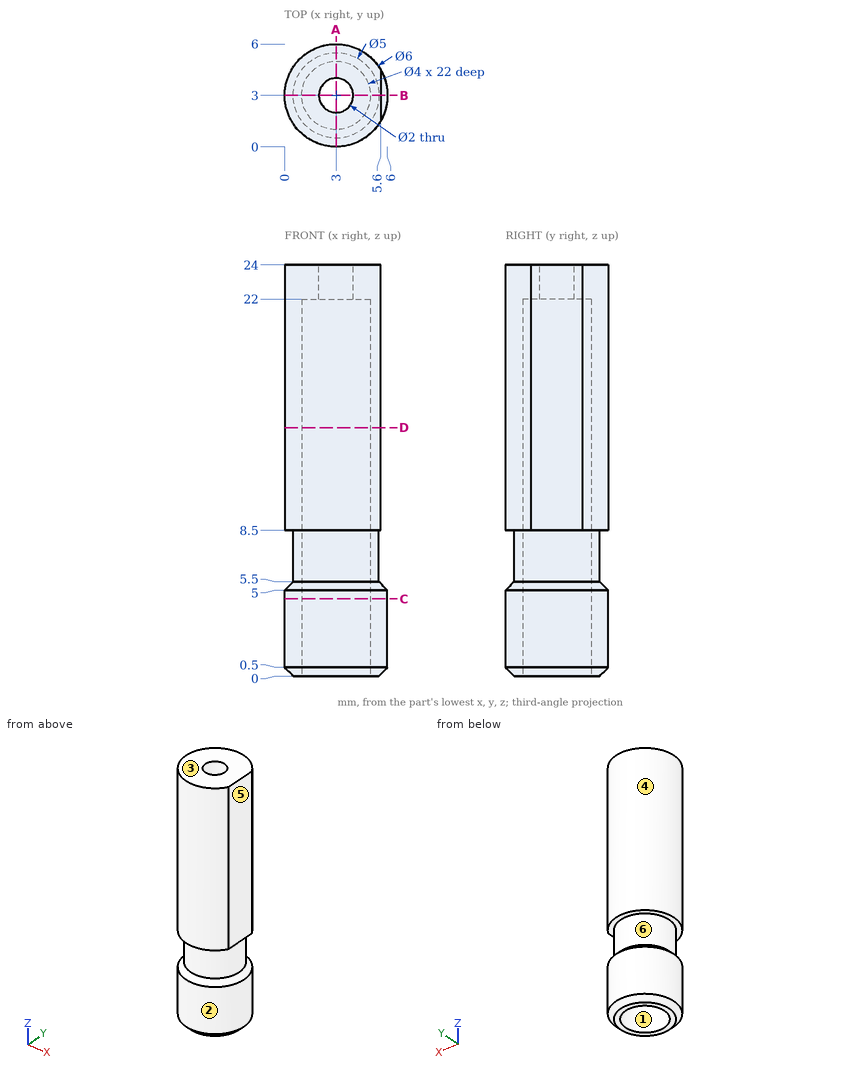
Geometry check sheet. Reference: drawing and pictorial views, mm from the part's lowest x, y, z. A direction names the side the tool comes from. Give positions to 0.01 mm unless a question says otherwise; leave off trailing zeros. Loops run counter-clockwise (first coordinate to the right, second up) from the corner with the lowest first, then second, coordinate; pieces in that order, holes last. Notation, with made-up numbers: M 82.5,24.5 L 121.5,24.5 A21 ccw 121.5,33.5 Z; hole C -7.75,25 d1. An arc over 180 degrees is marked long. Use a Markdown table: item, result. Add a question column.
Q1. Sectioned sample at D-D, the plane z = 14.5. Record the cut outline in (x, y).
Q2. Sectioned sample at A-A, the plane x = 3. Record the cut outline in (y, z).
Q3. Go/stop test with flat-tipped pins: pin 1 (1 mm diameter, centred on x = 4.5, z = 6, fed in from -Y); pin 2 (2.5 mm diameter, centred on y = 2.5, z = 16.5, fed in from +X). Record where each tip stops, or that it passes through.
Q4. Sectioned sample at C-C, the plane z = 4.5. Record the cut outline in (x, y), then the cut area to 3 significant figures.
Q5. Scan lines: line 1 along Y through (x, z) = (3, 23.05); line 2 along Y through (x, z) = (3, 15); line 3 along Z through (x, y) = (2.5, 2). Record each from-to range of solid material in increasing order. Write a range as [from, to].
Q6. Mould release check, pull along X, two halves, no side actions. Record for the marked faces 1, 2 and 3: pulls with the +X half, pulls with the -X half, needs draft (parallel to the pull), parting line crosses it, or undercut.
Q7. Tool access check on the marked faces 4, 5 and 6. Record the directions out of +Z, -Z, +X, -X, +Y, -Y that give a thin tool (end or side, any length) a straight path to the whole face; none if there is none.
Q8. Sectioned sample at B-B, the plane y = 3. Record the cut outline in (x, z).
Verdict:
| question | item | result |
|---|---|---|
| 1 | outline | M 5.6,1.5 L 5.6,4.5 A3 ccw long Z; hole C 3,3 d4 |
| 2 | outline | M 0,0.5 L 0.5,0 L 1,0 L 1,22 L 2,22 L 2,24 L 0,24 L 0,8.5 L 0.5,8.5 L 0.5,5.5 L 0,5 Z; M 4,22 L 5,22 L 5,0 L 5.5,0 L 6,0.5 L 6,5 L 5.5,5.5 L 5.5,8.5 L 6,8.5 L 6,24 L 4,24 Z |
| 3 | pin 1 | y = 0.71 |
| 3 | pin 2 | x = 5.6 |
| 4 | outline | C 3,3 d6; hole C 3,3 d4 |
| 4 | area | 15.7 mm^2 |
| 5 | line 1 | [0, 2], [4, 6] |
| 5 | line 2 | [0, 1], [5, 6] |
| 5 | line 3 | [22, 24] |
| 6 | face 1 | undercut |
| 6 | face 2 | parting line crosses it |
| 6 | face 3 | needs draft |
| 7 | face 4 | +Z, -Z |
| 7 | face 5 | +Z, +X, +Y, -Y |
| 7 | face 6 | none |
| 8 | outline | M 0,0.5 L 0.5,0 L 1,0 L 1,22 L 2,22 L 2,24 L 0,24 L 0,8.5 L 0.5,8.5 L 0.5,5.5 L 0,5 Z; M 4,22 L 5,22 L 5,0 L 5.5,0 L 6,0.5 L 6,5 L 5.5,5.5 L 5.5,8.5 L 5.6,8.5 L 5.6,24 L 4,24 Z |
